Source: CAD feature listing. Evaluate the final solid. Frame: model axes, mm. Face numbers are marked on the shaded views. A direction names the side the tool comes from. Round coordinates to 2 decimals unless told otherwise and drop trailing zeros. Order: outer loops, then holes, each group sorted by start corner. A loop starts at its lowest first (then second) coordinate and runs counter-clockwise, first axis right, second up. Notation, with made-up numbers: (82, 32) -> (102, 32) arc R27 cw to (102, 54) -> close; hole circle Ø4 at (37, -21). An arc over 180 degrees is marked (long way). Answer as CSV lines item,"result". Start each with the question number.
(1) Contact query for flat-ended pins moving along their axis: P1, Ø2, axis at x = -10.5, z = 2, coming from the -Y side; P2, Ø2, axis at x = 0, z = 4, coming from the -Y side; P3, Ø2, axis at x = -11.5, z = 3, coming from the +Y side; P4, Ø3, axis at x = -5.5, z = 2, coming from the +Y side. Output: stop coordinate, or through.
(2) Section query B-B (x = -2). Output: boundary loops of the cut face in (y, z).
(3) Pull-direction query (X, two-part tool) for the marked faces 1, 2 and 3; classes: +X half, -X half, draft (parallel to the pull), parting line (faces both ways), or undercut.
(4) Section query C-C (z = 3.5). Count the separate pieces of the cut face and the enclosed holes in it, plus the area to 3 significant figures.
(5) Line query: line 1 along Y through (x, z) = (-14, 6.5); line 2 along Y through (x, z) = (-8, 3.75); line 3 along Y through (x, z) = (7.75, 3.75). Output: solid intervals per line, ascending. Write a range as from..to.
(6) Section query D-D (y = -24.5). Output: boundary loops of the cut face in (x, z), plus the area to 3 significant figures.
(7) Section query A-A (x = 5.5). Output: boundary loops of the cut face in (y, z).
(8) Set-up query: the marked faces 4, 5 and 6. Return all of +Z, -Z, +X, -X, +Y, -Y with unobstructed straight access to the full face (end or side cutting, diameter ignored); none if empty.
```python
from build123d import *

# Parameters (mm, degrees)
F1_DEPTH      = 7
F2_W          = 6
F2_H          = 3
F3_DEPTH      = 7.001
F4_R          = 1.75
F5_DEPTH      = 5.001
F6_R          = 2
F7_DEPTH      = 4.251
F7_DEPTH_BACK = 45.6176002653


# Not quite as in the source:
# - a feature names something its author has since deleted; it is built from what else it names


with BuildPart() as f1:
    # F0 (on Top) → F1 (new body)
    with BuildSketch(Plane.XY):
        with BuildLine():
            ThreePointArc((-7.3654599313, -6), (-8.6701827743, -3.8830311175), (-9.3808315196, -1.5))
            Line((-9.3808315196, -1.5), (-15.4559988071, -1.5))
            Line((-15.4559988071, -1.5), (-15.4559988071, -6))
            Line((-15.4559988071, -6), (-7.3654599313, -6))
        make_face()
        with BuildLine():
            ThreePointArc((-4.5, 6), (3.3541019662, 6.7082039325), (7.5, 0))
            ThreePointArc((7.5, 0), (0.753817215, -7.4620211475), (-7.3484692283, -1.5))
            Line((-7.3484692283, -1.5), (-9.3808315196, -1.5))
            ThreePointArc((-9.3808315196, -1.5), (-8.6701827743, -3.8830311175), (-7.3654599313, -6))
            ThreePointArc((-7.3654599313, -6), (-1.8582019154, -9.3164953519), (4.5, -8.3666002653))
            ThreePointArc((4.5, -8.3666002653), (8.1547532152, -4.8733971724), (9.5, 0))
            ThreePointArc((9.5, 0), (3.1841899011, 8.9504711984), (-7.3654599313, 6))
            Line((-7.3654599313, 6), (-4.5, 6))
        make_face()
        with BuildLine():
            ThreePointArc((-7.3484692283, 1.5), (-6.3371173071, 4.0113519213), (-4.5, 6))
            Line((-4.5, 6), (-7.3654599313, 6))
            ThreePointArc((-7.3654599313, 6), (-8.6701827743, 3.8830311175), (-9.3808315196, 1.5))
            Line((-9.3808315196, 1.5), (-7.3484692283, 1.5))
        make_face()
        with BuildLine():
            ThreePointArc((-9.3808315196, 1.5), (-8.6701827743, 3.8830311175), (-7.3654599313, 6))
            Line((-7.3654599313, 6), (-15.4559988071, 6))
            Line((-15.4559988071, 6), (-15.4559988071, 1.5))
            Line((-15.4559988071, 1.5), (-9.3808315196, 1.5))
        make_face()
        with BuildLine():
            Line((9.5, -40.3666002653), (9.5, 0))
            ThreePointArc((9.5, 0), (8.1547532152, -4.8733971724), (4.5, -8.3666002653))
            Line((4.5, -8.3666002653), (4.5, -40.3666002653))
            Line((4.5, -40.3666002653), (9.5, -40.3666002653))
        make_face()
    extrude(amount=F1_DEPTH)

    # F2 (on face) → F3 (cut, through all)
    with BuildSketch(Plane.XY.offset(7)):
        with Locations((-11.4022340177, 3.75)):
            Rectangle(F2_W, F2_H)
    extrude(amount=-F3_DEPTH, mode=Mode.SUBTRACT)

    # F4 (on face) → F5 (cut, through all)
    with BuildSketch(Plane(origin=(4.5, 0, 0), x_dir=(0, -1, 0), z_dir=(-1, 0, 0))):
        with Locations((13.3666002653, 3.5)):
            Circle(F4_R)
        with Locations((37.3666002653, 3.5)):
            Circle(F4_R)
    extrude(amount=-F5_DEPTH, mode=Mode.SUBTRACT)

    # F6 (on face) → F7 (cut, two sides)
    with BuildSketch(Plane.XZ.offset(-5.25)) as f7_sk:
        with Locations((-11.4022340177, 3.5)):
            Circle(F6_R)
    extrude(amount=-F7_DEPTH, mode=Mode.SUBTRACT)
    extrude(f7_sk.sketch, amount=F7_DEPTH_BACK, mode=Mode.SUBTRACT)


solid = f1.part
```
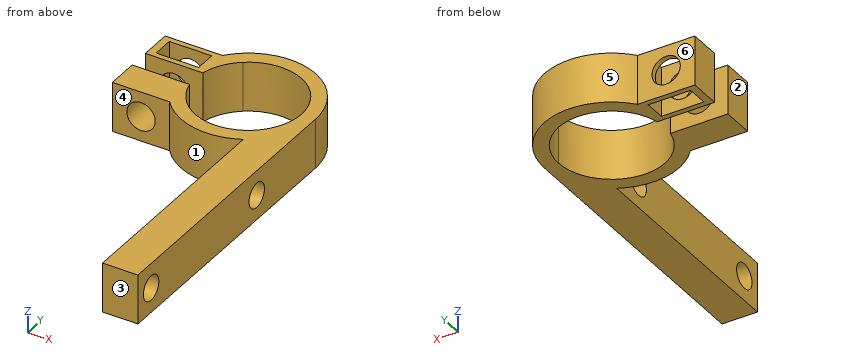
Answer block:
1,P1,"y = -6"
1,P2,"y = -9.5"
1,P3,"through"
1,P4,"y = 8.62"
2,outline,"(-9.29, 0) -> (-7.23, 0) -> (-7.23, 7) -> (-9.29, 7) -> close; (7.23, 0) -> (9.29, 0) -> (9.29, 7) -> (7.23, 7) -> close"
3,face 1,"undercut"
3,face 2,"-X half"
3,face 3,"draft"
4,separate pieces,"5"
4,enclosed holes,"0"
4,area,"257 mm2"
5,line 1,"-6..-1.5, 1.5..2.25, 5.25..6"
5,line 2,"-6..-1.5, 1.5..6"
5,line 3,"-40.37..-39.1, -35.63..-15.1, -11.63..5.49"
6,outline,"(4.5, 0) -> (9.5, 0) -> (9.5, 7) -> (4.5, 7) -> close"
6,area,"35.0 mm2"
7,outline,"(-40.37, 0) -> (-5.1, 0) -> (-5.1, 7) -> (-40.37, 7) -> close; (5.1, 0) -> (7.75, 0) -> (7.75, 7) -> (5.1, 7) -> close; hole circle Ø3.5 at (-37.37, 3.5); hole circle Ø3.5 at (-13.37, 3.5)"
8,face 4,"+Z, -Z, -X, -Y"
8,face 5,"+Z, -Z, +Y"
8,face 6,"+Z, -Z, -X, +Y"
